For this review, take the finished solid that the model builds, in its own axes (mm). A direction names the side the tool comes from. Round coordinates to 2 decimals unless told otherwise and drop trailing zeros. Write each loop counter-clockwise with the first axis right and the second up, starting at its lowest first coordinate (ties: lowest second). Pieces come first, ordered by that corner, then holes.
from build123d import *

# Parameters (mm, degrees)
SKETCH2_R           = 0.7
BOSS_EXTRUDE1_DEPTH = 2
FILLET1_R           = 1


with BuildPart() as part:
    # Sketch2 → Boss-Extrude1 (new body)
    # profile 1 of 16: a face of its own
    with BuildSketch(Plane(origin=(0, 0, 0), x_dir=(1, 0, 0), z_dir=(0, 1, 0))):
        with BuildLine():
            Line((-7.423854723, 0.808378324), (-9.191621676, 2.576145277))
            ThreePointArc((-9.191621676, 2.576145277), (-12.7, 0), (-9.191621676, -2.576145277))
            Line((-9.191621676, -2.576145277), (-7.423854723, -0.808378324))
            ThreePointArc((-7.423854723, -0.808378324), (-7.331143293, -0.408905706), (-7.3, 0))
            ThreePointArc((-7.3, 0), (-7.331143293, 0.408905706), (-7.423854723, 0.808378324))
        make_face()
        with Locations(Location((-10, 0, 0), (0, 0, 270))):
            Circle(SKETCH2_R, mode=Mode.SUBTRACT)
    # profile 2 of 16: a face of its own
    with BuildSketch(Plane(origin=(0, 0, 0), x_dir=(1, 0, 0), z_dir=(0, 1, 0))):
        with BuildLine():
            ThreePointArc((-0.808378324, 7.423854723), (-1.909188309, 8.090811691), (-2.576145277, 9.191621676))
            Line((-2.576145277, 9.191621676), (-9.191621676, 2.576145277))
            ThreePointArc((-9.191621676, 2.576145277), (-8.090811691, 1.909188309), (-7.423854723, 0.808378324))
            Line((-7.423854723, 0.808378324), (-0.808378324, 7.423854723))
        make_face()
    # profile 3 of 16: a face of its own
    with BuildSketch(Plane(origin=(0, 0, 0), x_dir=(1, 0, 0), z_dir=(0, 1, 0))):
        with BuildLine():
            ThreePointArc((2.7, 10), (-0.408905706, 12.668856707), (-2.576145277, 9.191621676))
            Line((-2.576145277, 9.191621676), (-0.808378324, 7.423854723))
            ThreePointArc((-0.808378324, 7.423854723), (0, 7.3), (0.808378324, 7.423854723))
            Line((0.808378324, 7.423854723), (2.576145277, 9.191621676))
            ThreePointArc((2.576145277, 9.191621676), (2.668856707, 9.591094294), (2.7, 10))
        make_face()
        with Locations(Location((0, 10, 0), (0, 0, 270))):
            Circle(SKETCH2_R, mode=Mode.SUBTRACT)
    # profile 4 of 16: a face of its own
    with BuildSketch(Plane(origin=(0, 0, 0), x_dir=(1, 0, 0), z_dir=(0, 1, 0))):
        with BuildLine():
            ThreePointArc((2.576145277, 9.191621676), (1.909188309, 8.090811691), (0.808378324, 7.423854723))
            Line((0.808378324, 7.423854723), (7.423854723, 0.808378324))
            ThreePointArc((7.423854723, 0.808378324), (8.090811691, 1.909188309), (9.191621676, 2.576145277))
            Line((9.191621676, 2.576145277), (2.576145277, 9.191621676))
        make_face()
    # profile 5 of 16: a face of its own
    with BuildSketch(Plane(origin=(0, 0, 0), x_dir=(1, 0, 0), z_dir=(0, 1, 0))):
        with BuildLine():
            Line((9.191621676, 2.576145277), (7.423854723, 0.808378324))
            ThreePointArc((7.423854723, 0.808378324), (7.3, 0), (7.423854723, -0.808378324))
            Line((7.423854723, -0.808378324), (9.191621676, -2.576145277))
            ThreePointArc((9.191621676, -2.576145277), (11.598026678, -2.176306673), (12.7, 0))
            ThreePointArc((12.7, 0), (11.598026678, 2.176306673), (9.191621676, 2.576145277))
        make_face()
        with Locations(Location((10, 0, 0), (0, 0, 270))):
            Circle(SKETCH2_R, mode=Mode.SUBTRACT)
    # profile 6 of 16: a face of its own
    with BuildSketch(Plane(origin=(0, 0, 0), x_dir=(1, 0, 0), z_dir=(0, 1, 0))):
        with BuildLine():
            ThreePointArc((9.191621676, -2.576145277), (8.090811691, -1.909188309), (7.423854723, -0.808378324))
            Line((7.423854723, -0.808378324), (0.808378324, -7.423854723))
            ThreePointArc((0.808378324, -7.423854723), (1.909188309, -8.090811691), (2.576145277, -9.191621676))
            Line((2.576145277, -9.191621676), (9.191621676, -2.576145277))
        make_face()
    # profile 7 of 16: a face of its own
    with BuildSketch(Plane(origin=(0, 0, 0), x_dir=(1, 0, 0), z_dir=(0, 1, 0))):
        with BuildLine():
            Line((-0.808378324, -7.423854723), (-2.576145277, -9.191621676))
            ThreePointArc((-2.576145277, -9.191621676), (-0.408905706, -12.668856707), (2.7, -10))
            ThreePointArc((2.7, -10), (2.668856707, -9.591094294), (2.576145277, -9.191621676))
            Line((2.576145277, -9.191621676), (0.808378324, -7.423854723))
            ThreePointArc((0.808378324, -7.423854723), (0, -7.3), (-0.808378324, -7.423854723))
        make_face()
        with Locations(Location((0, -10, 0), (0, 0, 270))):
            Circle(SKETCH2_R, mode=Mode.SUBTRACT)
    # profile 8 of 16: a face of its own
    with BuildSketch(Plane(origin=(0, 0, 0), x_dir=(1, 0, 0), z_dir=(0, 1, 0))):
        with BuildLine():
            ThreePointArc((-7.423854723, -0.808378324), (-8.090811691, -1.909188309), (-9.191621676, -2.576145277))
            Line((-9.191621676, -2.576145277), (-2.576145277, -9.191621676))
            ThreePointArc((-2.576145277, -9.191621676), (-1.909188309, -8.090811691), (-0.808378324, -7.423854723))
            Line((-0.808378324, -7.423854723), (-7.423854723, -0.808378324))
        make_face()
    # profile 9 of 16: a face of its own
    with BuildSketch(Plane(origin=(0, 0, 0), x_dir=(1, 0, 0), z_dir=(0, 1, 0))):
        with BuildLine():
            Line((-7.423854723, -0.808378324), (-9.191621676, -2.576145277))
            ThreePointArc((-9.191621676, -2.576145277), (-8.090811691, -1.909188309), (-7.423854723, -0.808378324))
        make_face()
    # profile 10 of 16: a face of its own
    with BuildSketch(Plane(origin=(0, 0, 0), x_dir=(1, 0, 0), z_dir=(0, 1, 0))):
        with BuildLine():
            ThreePointArc((-7.423854723, 0.808378324), (-8.090811691, 1.909188309), (-9.191621676, 2.576145277))
            Line((-9.191621676, 2.576145277), (-7.423854723, 0.808378324))
        make_face()
    # profile 11 of 16: a face of its own
    with BuildSketch(Plane(origin=(0, 0, 0), x_dir=(1, 0, 0), z_dir=(0, 1, 0))):
        with BuildLine():
            Line((-0.808378324, 7.423854723), (-2.576145277, 9.191621676))
            ThreePointArc((-2.576145277, 9.191621676), (-1.909188309, 8.090811691), (-0.808378324, 7.423854723))
        make_face()
    # profile 12 of 16: a face of its own
    with BuildSketch(Plane(origin=(0, 0, 0), x_dir=(1, 0, 0), z_dir=(0, 1, 0))):
        with BuildLine():
            Line((2.576145277, 9.191621676), (0.808378324, 7.423854723))
            ThreePointArc((0.808378324, 7.423854723), (1.909188309, 8.090811691), (2.576145277, 9.191621676))
        make_face()
    # profile 13 of 16: a face of its own
    with BuildSketch(Plane(origin=(0, 0, 0), x_dir=(1, 0, 0), z_dir=(0, 1, 0))):
        with BuildLine():
            ThreePointArc((9.191621676, 2.576145277), (8.090811691, 1.909188309), (7.423854723, 0.808378324))
            Line((7.423854723, 0.808378324), (9.191621676, 2.576145277))
        make_face()
    # profile 14 of 16: a face of its own
    with BuildSketch(Plane(origin=(0, 0, 0), x_dir=(1, 0, 0), z_dir=(0, 1, 0))):
        with BuildLine():
            Line((9.191621676, -2.576145277), (7.423854723, -0.808378324))
            ThreePointArc((7.423854723, -0.808378324), (8.090811691, -1.909188309), (9.191621676, -2.576145277))
        make_face()
    # profile 15 of 16: a face of its own
    with BuildSketch(Plane(origin=(0, 0, 0), x_dir=(1, 0, 0), z_dir=(0, 1, 0))):
        with BuildLine():
            ThreePointArc((2.576145277, -9.191621676), (1.909188309, -8.090811691), (0.808378324, -7.423854723))
            Line((0.808378324, -7.423854723), (2.576145277, -9.191621676))
        make_face()
    # profile 16 of 16: a face of its own
    with BuildSketch(Plane(origin=(0, 0, 0), x_dir=(1, 0, 0), z_dir=(0, 1, 0))):
        with BuildLine():
            ThreePointArc((-0.808378324, -7.423854723), (-1.909188309, -8.090811691), (-2.576145277, -9.191621676))
            Line((-2.576145277, -9.191621676), (-0.808378324, -7.423854723))
        make_face()
    extrude(amount=BOSS_EXTRUDE1_DEPTH)

    # Fillet1
    fillet1_edges = [part.edges().sort_by_distance(p)[0] for p in [
        (-2.576145277, 1, 9.191621676),
        (-9.191621676, 1, 2.576145277),
        (-9.191621676, 1, -2.576145277),
        (-2.576145277, 1, -9.191621676),
        (2.576145277, 1, -9.191621676),
        (9.191621676, 1, -2.576145277),
        (9.191621676, 1, 2.576145277),
        (2.576145277, 1, 9.191621676),
        (-0.808378324, 1, -7.423854723),
        (-7.423854723, 1, -0.808378324),
        (-7.423854723, 1, 0.808378324),
        (-0.808378324, 1, 7.423854723),
        (0.808378324, 1, 7.423854723),
        (7.423854723, 1, 0.808378324),
        (7.423854723, 1, -0.808378324),
        (0.808378324, 1, -7.423854723),
    ]]
    fillet(fillet1_edges, radius=FILLET1_R)


solid = part.part
(1) We need section A-A, the plane x = 10. Give the boundary of the cut face in (y, z).
Geometry check:
outline: (0, -2.7) - (2, -2.7) - (2, -0.7) - (0, -0.7) - close; (0, 0.7) - (2, 0.7) - (2, 2.7) - (0, 2.7) - close
(2) For faces 4 (the face through (9.2, 1.01, -2.72)), 5 (the face through (7.28, 1.01, 0.81)), list the 3-axis set-ups (+Z, -Z, +X, -X, +Y, -Y) from which the entire face can be reached by the end or side of a thin tool; tool diameter is ignored.
Geometry check:
face 4: -Z, +Y, -Y
face 5: +Y, -Y
(3) For pin 1 Ø4 at (x, z) = (4, 8) entering from +Y; pin 2 Ø1.1 at (x, z) = (10, 0) entering from -Y, all flat-tipped, find the tip position at first contact; note any pin that passes through.
Geometry check:
pin 1: stops at y = 2
pin 2: passes through
(4) For line 1 along X through (y, z) = (0.95, 0); line 2 along X through (y, z) = (1.15, 10); line 3 along X through (y, z) = (0.85, -2), list the stretches that pass through material, from the lowest coordinate up.
Geometry check:
line 1: x = -12.7 to -10.7, -9.3 to -7.3, 7.3 to 9.3, 10.7 to 12.7
line 2: x = -2.7 to -0.7, 0.7 to 2.7
line 3: x = -11.81 to -6.23, 6.23 to 11.81
(5) We need section C-C, the plane z = -6.5. Give the boundary of the cut face in (x, y).
Geometry check:
outline: (-5.27, 0) - (-1.73, 0) - (-1.73, 2) - (-5.27, 2) - close; (1.73, 0) - (5.27, 0) - (5.27, 2) - (1.73, 2) - close
(6) Mouldability with a two-part tool opening along Z and no side actions: class faces 1 (the face through (-9.19, 1.01, 2.72)), 2 (the face through (-5.843, 0.986, -5.925)), 3 (the face through (-7.28, 1.01, 0.81)) as pulls with the +Z half, pulls with the -Z half, needs draft (parallel to the pull), parting line crosses it, or undercut.
Geometry check:
face 1: pulls with the +Z half
face 2: pulls with the -Z half
face 3: undercut
(7) We need section B-B, the plane x = 0. Give the boundary of the cut face in (y, z).
Geometry check:
outline: (0, -12.7) - (2, -12.7) - (2, -10.7) - (0, -10.7) - close; (0, -9.3) - (2, -9.3) - (2, -7.3) - (0, -7.3) - close; (0, 7.3) - (2, 7.3) - (2, 9.3) - (0, 9.3) - close; (0, 10.7) - (2, 10.7) - (2, 12.7) - (0, 12.7) - close
(8) We need section D-D, the plane y = 0.95. State how many separate pieces and enclosed holes the cut face has, and give its area (3 significant figures).
Geometry check:
separate pieces: 1
enclosed holes: 5
area: 176 mm2
